Source: CAD feature listing. Evaluate the final solid. Frame: model axes, mm. A direction names the side the tool comes from. Give positions to 0.01 mm unless a question says otherwise; leave off trailing zeros. Write each loop counter-clockwise with the first axis right and the second up, starting at its lowest first coordinate (ties: lowest second). Pieces come first, ordered by that corner, then holes. Notation, with made-up numbers: M -23.5,-7.5 L -8.5,-7.5 A17 ccw -8.5,18.5 Z; hole C 35.5,45 d11. An arc over 180 degrees is marked long. Use CSV: the item, a comma, the result in double quotes. Start each with the question number.
from build123d import *

# Parameters (mm, degrees)
SKETCH_1_W      = 91.44
SKETCH_1_H      = 25.4
SKETCH_1_R      = 1.6
EXTRUDE_1_DEPTH = 1.6
SKETCH_2_W      = 15.3
SKETCH_2_H      = 22.8
EXTRUDE_2_DEPTH = 5
SKETCH_3_W      = 17.7
SKETCH_3_H      = 22.8
EXTRUDE_3_DEPTH = 10


with BuildPart() as part:
    # 草图1 → 凸台-拉伸1 (new body)
    with BuildSketch(Plane(origin=(0, 0, 0), x_dir=(1, 0, 0), z_dir=(0, 1, 0))):
        Rectangle(SKETCH_1_W, SKETCH_1_H)
        with Locations(Location((-43.18, 10.16, 0), (0, 0, 270))):
            Circle(SKETCH_1_R, mode=Mode.SUBTRACT)
        with Locations(Location((43.18, 10.16, 0), (0, 0, 90))):
            Circle(SKETCH_1_R, mode=Mode.SUBTRACT)
        with Locations(Location((43.18, -10.16, 0), (0, 0, 270))):
            Circle(SKETCH_1_R, mode=Mode.SUBTRACT)
        with Locations(Location((-43.18, -10.16, 0), (0, 0, 90))):
            Circle(SKETCH_1_R, mode=Mode.SUBTRACT)
    extrude(amount=EXTRUDE_1_DEPTH)

    # 草图2 → 凸台-拉伸2 (add)
    with BuildSketch(Plane(origin=(0, 1.6, 0), x_dir=(1, 0, 0), z_dir=(0, 1, 0))):
        with Locations((-31.75, 0)):
            Rectangle(SKETCH_2_W, SKETCH_2_H)
    extrude(amount=EXTRUDE_2_DEPTH)

    # 草图3 → 凸台-拉伸3 (add)
    with BuildSketch(Plane(origin=(0, 1.6, 0), x_dir=(1, 0, 0), z_dir=(0, 1, 0))):
        with Locations((20.25, 0)):
            Rectangle(SKETCH_3_W, SKETCH_3_H)
    extrude(amount=EXTRUDE_3_DEPTH)


solid = part.part
1. Access query for faces 5 (the flat face through (29.1, 7, 0)), 6 (the flat face through (11.4, 7, 0)), 7 (the flat face through (-32, 6.6, 0)), 8 (the flat face through (20, 7, 11.4)). Directions: +Z, -Z, +X, -X, +Y, -Y. A direction counts if a zero-diameter tool reaches every point of the face in a straight line with its end or side. Return the directions, or none.
2. Section C-C on z = 3.75. Return loops of the section in (x, y).
3. Line query: probe 1 along X at (y, z) = (0.75, -10.16); probe 2 along X at (y, z) = (3.75, -10.25); probe 3 along Z at (x, y) = (17.5, 6). Output: solid intervals per line, ascending.
4. Section A-A on z = 10.16. Return loops of the section in (x, y).
5. Section B-B on x = 43.18. Return loops of the section in (y, z), then the cut area to 3 significant figures.
6. First-contact query: pin 1 (3 mm diameter, centred on x = 18, y = 8, fed in from -Z); pin 2 (6 mm diameter, centred on y = 7, z = -5.5, fed in from +X); pin 3 (3 mm diameter, centred on x = -21.5, z = 7.5, fed in from +Y); pin 4 (2.5 mm diameter, centred on x = 43.18, z = -10.16, fed in from -Y). Flat tips, straight axial feed; report the tip coordinate or a pass-through.
7. Pull-direction query (Z, two-part tool) for faces 1 (the cylindrical face through (-44.6, 0.79, -9.42)), 2 (the cylindrical face through (44.15, 0.79, -8.89)), 3 (the flat face through (20, 7, -11.4)), 4 (the flat face through (-39.4, 4, 0)); classes: released by +Z, released by -Z, zero draft, split by the parting line, or undercut.
8. Section D-D on x = -8.5. Return loops of the section in (y, z).
Resolved:
1,face 5,"+Z, -Z, +X, +Y"
1,face 6,"+Z, -Z, +Y"
1,face 7,"+Z, -Z, -X, +Y"
1,face 8,"+Z, +X, -X, +Y"
2,outline,"M -45.72,0 L 45.72,0 L 45.72,1.6 L 29.1,1.6 L 29.1,11.6 L 11.4,11.6 L 11.4,1.6 L -24.1,1.6 L -24.1,6.6 L -39.4,6.6 L -39.4,1.6 L -45.72,1.6 Z"
3,probe 1,"x = -45.72 to -44.78, -41.58 to 41.58, 44.78 to 45.72"
3,probe 2,"x = -39.4 to -24.1, 11.4 to 29.1"
3,probe 3,"z = -11.4 to 11.4"
4,outline,"M -45.72,0 L -44.78,0 L -44.78,1.6 L -45.72,1.6 Z; M -41.58,0 L 41.58,0 L 41.58,1.6 L 29.1,1.6 L 29.1,11.6 L 11.4,11.6 L 11.4,1.6 L -24.1,1.6 L -24.1,6.6 L -39.4,6.6 L -39.4,1.6 L -41.58,1.6 Z; M 44.78,0 L 45.72,0 L 45.72,1.6 L 44.78,1.6 Z"
5,outline,"M 0,-12.7 L 1.6,-12.7 L 1.6,-11.76 L 0,-11.76 Z; M 0,-8.56 L 1.6,-8.56 L 1.6,8.56 L 0,8.56 Z; M 0,11.76 L 1.6,11.76 L 1.6,12.7 L 0,12.7 Z"
5,area,"30.4 mm2"
6,pin 1,"stops at z = -11.4"
6,pin 2,"stops at x = 29.1"
6,pin 3,"stops at y = 1.6"
6,pin 4,"passes through"
7,face 1,"undercut"
7,face 2,"undercut"
7,face 3,"released by -Z"
7,face 4,"zero draft"
8,outline,"M 0,-12.7 L 1.6,-12.7 L 1.6,12.7 L 0,12.7 Z"
